Job drawing, mm, ordinate dimensions from the low corner. One solid piece. Round coordinates to 2 decimals unless told otherwise and drop trailing zeros. Loops run counter-clockwise (first coordinate to the right, second up) from the corner with the lowest first, then second, coordinate; pieces in that order, holes last. Notation, with made-up numbers: M 47,83 L 88,83 A18 cw 88,105 Z; hole C -7,24 d7. An arc over 180 degrees is marked long. Write each question's results on one line, items separated by ' | '. Start each with the question number.
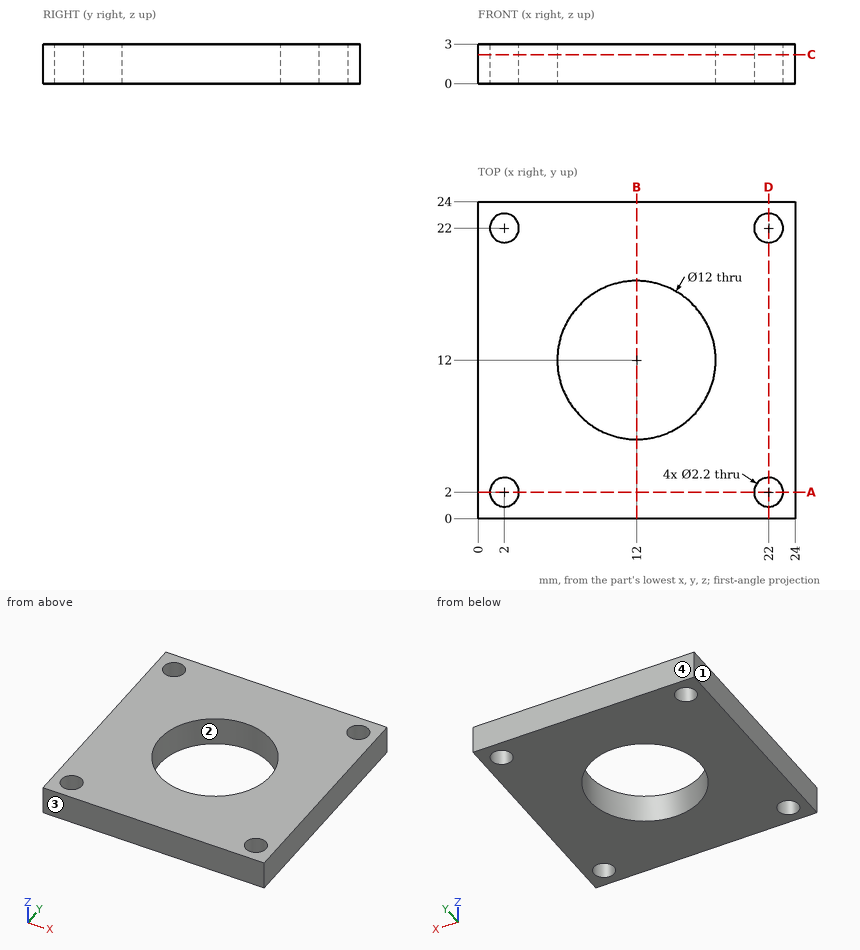
Item 1: Saw through at A-A, the plane y = 2. Give the cut face in (x, z).
Item 2: Saw through at C-C, the plane z = 2.2. Give the cut face in (x, y), then the cut area to 3 significant figures.
Item 3: Drill centre lines: line 1 along X through (y, z) = (22, 1.15); line 2 along X through (y, z) = (12, 1.95). Where is each one in solid material? Low to high. Write a range as [from, to].
Item 4: Mould opens along Y. For the marked faces 1, 2, 3 and 4 say: released by +Y, released by -Y, zero draft, split by the parting line, or undercut.
Item 5: Drop a flat-ended pin along its axis: pin 1 (1 mm diameter, centred on x = 17, z = 2, fed in from -Y). Give the stop position or say it passes through.
Item 6: Saw through at B-B, the plane x = 12. Give the cut face in (y, z).
Working result:
1) outline: M 0,0 L 0.9,0 L 0.9,3 L 0,3 Z; M 3.1,0 L 20.9,0 L 20.9,3 L 3.1,3 Z; M 23.1,0 L 24,0 L 24,3 L 23.1,3 Z
2) outline: M 0,0 L 24,0 L 24,24 L 0,24 Z; hole C 2,2 d2.2; hole C 2,22 d2.2; hole C 12,12 d12; hole C 22,2 d2.2; hole C 22,22 d2.2 | area: 448 mm²
3) line 1: x = [0, 0.9], [3.1, 20.9], [23.1, 24] | line 2: x = [0, 6], [18, 24]
4) face 1: zero draft | face 2: undercut | face 3: released by -Y | face 4: released by +Y
5) pin 1: stops at y = 0
6) outline: M 0,0 L 6,0 L 6,3 L 0,3 Z; M 18,0 L 24,0 L 24,3 L 18,3 Z
